Work out the finished part from the listing and answer in its coordinate system (mm). Face numbers are marked on the shaded views. A direction names the side the tool comes from. Round coordinates to 2 decimals unless told otherwise and drop trailing zeros. Use CSV: the item, a comma, the result in double quotes.
from build123d import *

# Parameters (mm, degrees)
SKETCH1_W               = 30
SKETCH1_H               = 15
BOSS_EXTRUDE1_DEPTH     = 5.5
CUT_EXTRUDE2_DEPTH      = 18.649362595
CUT_EXTRUDE2_DEPTH_BACK = 18.649362595
SKETCH2_W               = 0.5
SKETCH2_H               = 0.2
SKETCH5_W               = 9.2
SKETCH5_H               = 5.5
CUT_EXTRUDE4_DEPTH      = 1.6
SKETCH7_R               = 6.5
CUT_EXTRUDE6_DEPTH      = 1.75
FILLET1_R               = 1


with BuildPart() as part:
    # Sketch1 → Boss-Extrude1 (new body)
    with BuildSketch(Plane(origin=(0, 0, 0), x_dir=(1, 0, 0), z_dir=(0, 1, 0))):
        Rectangle(SKETCH1_W, SKETCH1_H)
    extrude(amount=BOSS_EXTRUDE1_DEPTH)

    # Sketch2 → Cut-Extrude2 (cut, two sides: drawn at the far end of the back side and taken through both)
    with BuildSketch(Plane(origin=(0, 0, 0), x_dir=(0, 0, -1), z_dir=(1, 0, 0)).offset(-CUT_EXTRUDE2_DEPTH_BACK)):
        with Locations((-5.75, 5.4)):
            Rectangle(SKETCH2_W, SKETCH2_H)
        with Locations((-3.75, 5.4)):
            Rectangle(SKETCH2_W, SKETCH2_H)
        with Locations((-1.75, 5.4)):
            Rectangle(SKETCH2_W, SKETCH2_H)
        with Locations((0.25, 5.4)):
            Rectangle(SKETCH2_W, SKETCH2_H)
        with Locations((2.25, 5.4)):
            Rectangle(SKETCH2_W, SKETCH2_H)
        with Locations((4.25, 5.4)):
            Rectangle(SKETCH2_W, SKETCH2_H)
        with Locations((6.25, 5.4)):
            Rectangle(SKETCH2_W, SKETCH2_H)
    extrude(amount=CUT_EXTRUDE2_DEPTH + CUT_EXTRUDE2_DEPTH_BACK, mode=Mode.SUBTRACT)

    # Sketch8 → Cut-Revolve1 (revolve, cut)
    with BuildSketch(Plane.XY.offset(4), mode=Mode.PRIVATE) as cut_revolve1_sk:
        Polygon((10.25, 0), (10.25, 3), (9, 3.721687836), (9, 0), align=None)
    cut_revolve1 = revolve(cut_revolve1_sk.sketch.rotate(Axis((9, 0, 4), (0, 1, 0)), 90), axis=Axis((9, 0, 4), (0, 1, 0)), mode=Mode.SUBTRACT)

    # Mirror1: Cut-Revolve1 across plane
    add(cut_revolve1.mirror(Plane.XY), mode=Mode.SUBTRACT)

    # Mirror2: Cut-Revolve1 across plane
    add(cut_revolve1.mirror(Plane(origin=(0, 0, 0), x_dir=(0, 0, 1), z_dir=(1, 0, 0))), mode=Mode.SUBTRACT)

    # Mirror2 copy 1 sketch → Mirror2 copy 1 (revolve, cut)
    with BuildSketch(Plane(origin=(0, 0, -4), x_dir=(-1, 0, 0), z_dir=(0, 0, -1))):
        Polygon((10.25, 0), (10.25, 3), (9, 3.721687836), (9, 0), align=None)
    revolve(axis=Axis((-9, 0, -4), (0, 1, 0)), mode=Mode.SUBTRACT)

    # Sketch5 → Cut-Extrude4 (cut)
    with BuildSketch(Plane(origin=(-15, 0, 0), x_dir=(0, 0, -1), z_dir=(1, 0, 0))):
        with Locations((-0.5, 2.75)):
            Rectangle(SKETCH5_W, SKETCH5_H)
    extrude(amount=CUT_EXTRUDE4_DEPTH, mode=Mode.SUBTRACT)

    # Sketch9 → Cut-Revolve2 (revolve, cut)
    with BuildSketch(Plane.XY):
        Polygon((-15, 2.5), (-7.678312164, 2.5), (-8.4, 3.75), (-15, 3.75), align=None)
    revolve(axis=Axis((-15, 2.5, 0), (-1, 0, 0)), mode=Mode.SUBTRACT)

    # Sketch7 → Cut-Extrude6 (cut)
    with BuildSketch(Plane.XZ):
        with Locations((17.59, 0)):
            Circle(SKETCH7_R)
    extrude(amount=-CUT_EXTRUDE6_DEPTH, mode=Mode.SUBTRACT)

    # Fillet1
    fillet1_edges = [part.edges().sort_by_distance(p)[0] for p in [
        (-15, 2.75, -7.5),
        (15, 2.75, -7.5),
        (15, 2.75, 7.5),
        (-15, 2.75, 7.5),
    ]]
    fillet(fillet1_edges, radius=FILLET1_R - 0.0001)  # a hair under: the kernel refuses the full size


solid = part.part
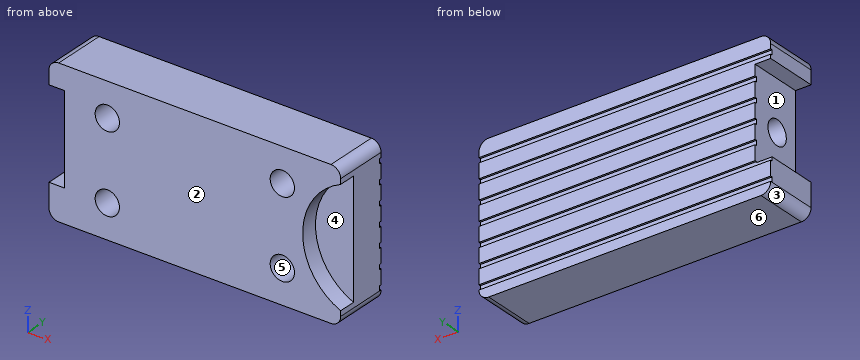
(1) The mould has two halves that part along Z. Classify the marked faces 1, 2, 3 and 4: released by +Z, released by -Z, zero draft, split by the parting line, or undercut.
Findings below:
face 1,"undercut"
face 2,"zero draft"
face 3,"released by -Z"
face 4,"undercut"
(2) Find the intervals of material crossed by L1, parallel to X at y = 1.9, z = 4; L2, parallel to X at y = 0.4, z = 4.75; L3, parallel to Z at x = -10.95, y = 2.5, in increasing order. Write a range as from..to.
Findings below:
L1,"x = -13.4..-10.25, -7.75..7.75, 10.25..15"
L2,"x = -13.4..-10, -8..8, 10..13.15"
L3,"z = -7.5..-1.25, 1.25..7.5"
(3) For the marked faces 5 and 6, determine the directions among +Z, -Z, +X, -X, +Y, -Y from which every point of the face is accessible in a straight line to the end or side of a thin tool.
Findings below:
face 5,"-Y"
face 6,"-Z, +X, -X, +Y, -Y"
